Answer from the drawing. Dimensions are ordinates in mm from the lowest x, y and z of the part. Round coordinates to 2 decimals unless told otherwise and drop trailing zeros. Loops run counter-clockwise (first coordinate to the right, second up) from the corner with the lowest first, then second, coordinate; pieces in that order, holes last. Notation, with made-up numbers: M 5.25,9 L 41.25,9 A13 cw 41.25,16 Z; hole C 56,16.25 d1. An arc over 180 degrees is marked long. One line per item, written item: value.
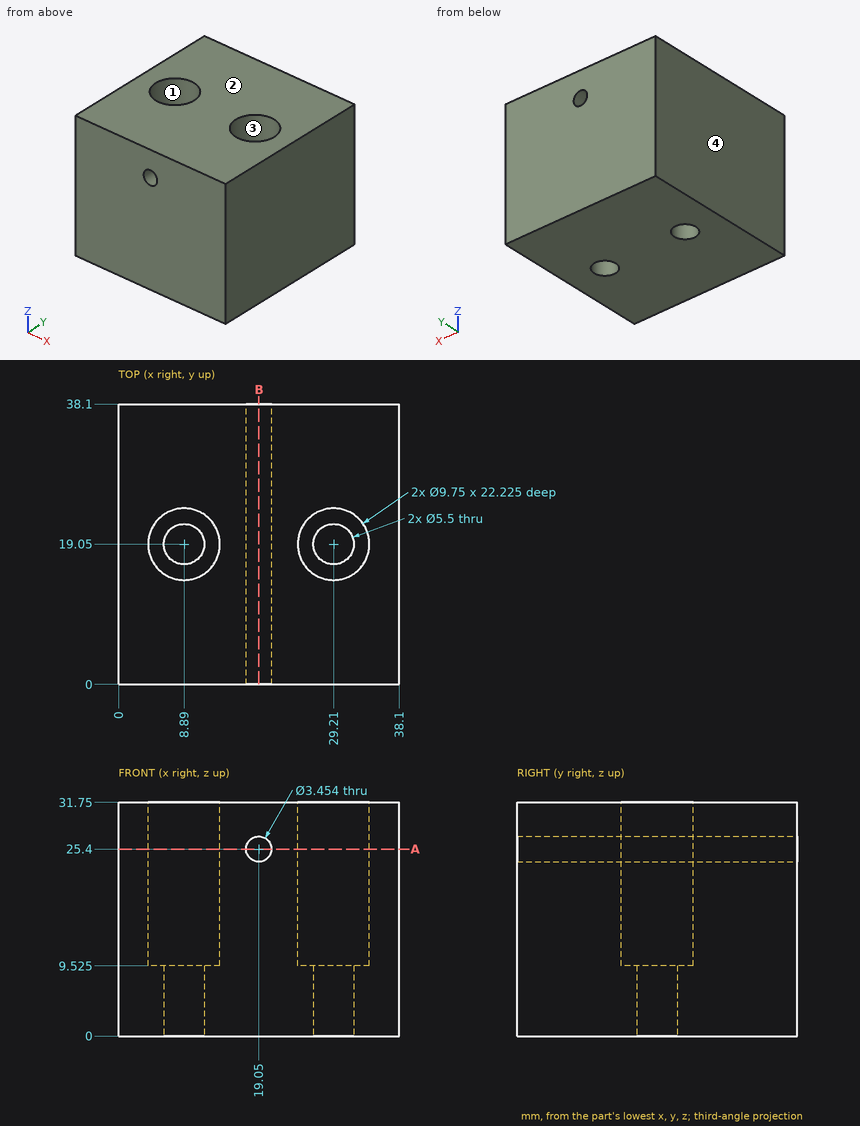
1) The mould has two halves that part along X. Classify the marked faces 1, 2, 3 and 4: +X half, -X half, draft (parallel to the pull), parting line (faces both ways), or undercut.
Check values:
face 1: undercut
face 2: draft
face 3: undercut
face 4: -X half
2) Find section A-A (z = 25.4). Give the number of separate pieces and of enclosed holes in the cut face, then the cut area to 3 significant figures.
Check values:
separate pieces: 2
enclosed holes: 2
area: 1,170 mm2
3) Each of these flat-tipped pins is pushed along its axis until it touches: pin 1 (3.5 mm diameter, centred on x = 8.89, y = 19.05, fed in from -Z); pin 2 (3 mm diameter, centred on x = 31, y = 19.5, fed in from +Z) (3 decimals). Where does it stop, or does it pass through?
Check values:
pin 1: through
pin 2: z = 9.525
4) Find the intervals of material crossed by probe 1 along X at (y, z) = (19, 19) (1 decimal); probe 2 along Z at (x, y) = (19, 25); probe 3 along X at (y, z) = (12, 25.5) (1 decimal), in increasing order. Write a range as from..to.
Check values:
probe 1: 0..4, 13.8..24.3, 34.1..38.1
probe 2: 0..23.67, 27.13..31.75
probe 3: 0..17.3, 20.8..38.1
5) Find section B-B (x = 19.05). Give the vertices of the cut face in (y, z), then the cut area to 3 significant figures.
Check values:
outline: M 0,0 L 38.1,0 L 38.1,23.67 L 0,23.67 Z; M 0,27.13 L 38.1,27.13 L 38.1,31.75 L 0,31.75 Z
area: 1,080 mm2
